Check sheet for the modelled part. Datum: model origin and axes. Units: mm. Face numbers are marked on the shaded views. Round coordinates to 2 decimals unless told otherwise and drop trailing zeros. Order: outer loops, then holes, each group sorted by start corner. A loop starts at its lowest first (then second) coordinate and runs counter-clockwise, first axis right, second up.
Q1. Scan lines: probe 1 along Z at (x, y) = (0, 5.5) (3 decimals); probe 2 along X at (y, z) = (8.5, 0.5); probe 3 along X at (y, z) = (4, 2.25). Record each from-to range of solid material in increasing order.
Q2. Cross-section at C-C on y = 2.75. Record the cut outline in (x, z) (3 decimals), then the cut area to 3 significant figures.
Q3. Cross-section at B-B on z = 0. Record the cut outline in (x, y) (3 decimals).
Q4. Cross-section at A-A on x = 0. Record the cut outline in (y, z) (3 decimals).
Q5. Depth check by flat-ended pin: P1, Ø1.5, axis at x = 4.5, y = 3.5, coming from the -Z side; P2, Ø1, axis at x = 0.5, z = -1, coming from the +Y side; P3, Ø6, axis at y = 7, z = -1, coming from the -X side (3 decimals); P4, Ø6, axis at y = 3.5, z = -6, coming from the +X side. Enter the tip coordinate at first touch or a pass-through.
Q6. Mould release check, pull along X, two halves, no side actions. Record for the marked faces 1, 2 and 3: +X half, -X half, draft (parallel to the pull), parting line (faces both ways), or undercut.
Q7. Cross-section at D-D on z = -6. Record the cut outline in (x, y), then the cut area to 3 significant figures.
from build123d import *

# Parameters (mm, degrees)
SKETCH2_R               = 9.525
BOSS_EXTRUDE1_DEPTH     = 1
M5_CLEARANCE_HOLE1_D    = 5.5
CUT_EXTRUDE1_DEPTH      = 1
CUT_EXTRUDE1_DEPTH_BACK = 2
SKETCH9_R               = 9.525
SKETCH9_R_2             = 2.75
BOSS_EXTRUDE2_DEPTH     = 10


with BuildPart() as part:
    # Sketch2 → Boss-Extrude1 (new body)
    with BuildSketch(Plane(origin=(0, 0, 0), x_dir=(1, 0, 0), z_dir=(0, 1, 0))):
        Circle(SKETCH2_R)
    extrude(amount=BOSS_EXTRUDE1_DEPTH)

    # M5 Clearance Hole1 (through all)
    with Locations(Plane(origin=(0, 1, 0), x_dir=(1, 0, 0), z_dir=(0, 1, 0))):
        with Locations((0, 0)):
            Hole(M5_CLEARANCE_HOLE1_D / 2)

    # Sketch7 → Cut-Extrude1 (cut, two sides)
    with BuildSketch(Plane(origin=(0, 1, 0), x_dir=(1, 0, 0), z_dir=(0, 1, 0))) as cut_extrude1_sk:
        Polygon((3.063849251, 9.018783331), (-3.927822903, 8.677432353), (-3.960317229, 9.342992692), (3.031354925, 9.68434367), align=None)
    extrude(amount=CUT_EXTRUDE1_DEPTH, mode=Mode.SUBTRACT)
    extrude(cut_extrude1_sk.sketch, amount=-CUT_EXTRUDE1_DEPTH_BACK, mode=Mode.SUBTRACT)

    # Sketch9 → Boss-Extrude2 (add)
    with BuildSketch(Plane.XZ):
        Circle(SKETCH9_R)
        Circle(SKETCH9_R_2, mode=Mode.SUBTRACT)
    extrude(amount=-BOSS_EXTRUDE2_DEPTH)


solid = part.part
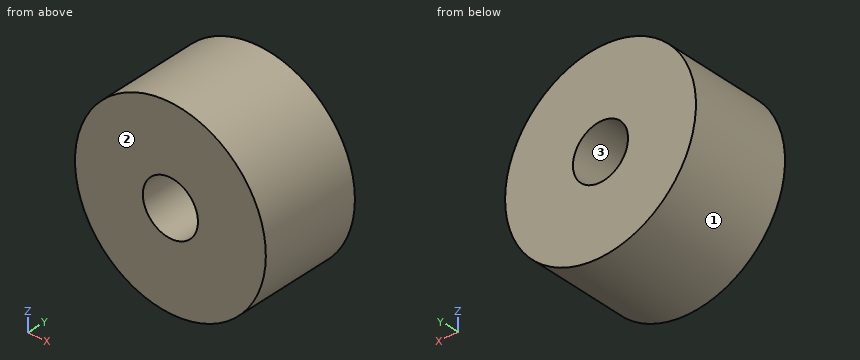
Results found:
1. probe 1: z = -9.525 to -2.75, 2.75 to 9.525
1. probe 2: x = -9.51 to -2.7, 2.7 to 9.51
1. probe 3: x = -9.26 to -1.58, 1.58 to 9.26
2. outline: circle Ø19.05 at (0, 0); hole circle Ø5.5 at (0, 0)
2. area: 261 mm2
3. outline: (-9.525, 0) - (-2.75, 0) - (-2.75, 10) - (-9.525, 10) - close; (2.75, 0) - (9.525, 0) - (9.525, 10) - (2.75, 10) - close
4. outline: (0, -9.525) - (10, -9.525) - (10, -2.75) - (0, -2.75) - close; (0, 2.75) - (10, 2.75) - (10, 9.525) - (0, 9.525) - close
5. P1: stops at z = -8.76
5. P2: passes through
5. P3: stops at x = -9.525
5. P4: stops at x = 9.04
6. face 1: parting line
6. face 2: draft
6. face 3: undercut
7. outline: (-7.4, 0) - (7.4, 0) - (7.4, 10) - (-7.4, 10) - close
7. area: 148 mm2
